from build123d import *

# Parameters (mm, degrees)
SCHIZZO1_W                     = 28
SCHIZZO1_H                     = 25
BASE_FLANGIA1_DEPTH            = 2
BORDO_FLANGIA1_STRIP_W         = 9.4732
BORDO_FLANGIA1_STRIP_H         = 2
BORDO_FLANGIA1_STRIP_CUT_DEPTH = 25
BORDO_FLANGIA1_DEPTH           = 25
SCHIZZO3_R                     = 4
SCHIZZO3_R_2                   = 1.5
TAGLIO_ESTRUSIONE1_DEPTH       = 40.714606885
SCHIZZO4_R                     = 1.5
SCHIZZO4_R_2                   = 4
TAGLIO_ESTRUSIONE2_DEPTH       = 47.917480751


# Sheet-metal steps are written as plain solids
with BuildPart() as part:
    # Schizzo1 → Base-Flangia1 (new body)
    with BuildSketch(Plane(origin=(0, 0, 0), x_dir=(1, 0, 0), z_dir=(0, 1, 0))):
        Rectangle(SCHIZZO1_W, SCHIZZO1_H)
    extrude(amount=BASE_FLANGIA1_DEPTH)

    # Bordo-Flangia1 strip (across the edge) → Bordo-Flangia1 strip cut (cut)
    with BuildSketch(Plane(origin=(-14, 2, -12.5), x_dir=(1, 0, 0), z_dir=(0, 0, 1))):
        with Locations((-2, -1)):
            Rectangle(BORDO_FLANGIA1_STRIP_W, BORDO_FLANGIA1_STRIP_H)
    extrude(amount=BORDO_FLANGIA1_STRIP_CUT_DEPTH, mode=Mode.SUBTRACT)

    # Bordo-Flangia1 section (across the edge) → Bordo-Flangia1 (add)
    with BuildSketch(Plane(origin=(-14, 2, -12.5), x_dir=(1, 0, 0), z_dir=(0, 0, 1))):
        with BuildLine():
            Line((0, 0.7366), (0, 35))
            Line((0, 35), (2, 35))
            Line((2, 35), (2, 0.7366))
            ThreePointArc((2, 0.7366), (2.215745145, 0.215745145), (2.7366, 0))
            Line((2.7366, 0), (2.7366, -2))
            ThreePointArc((2.7366, -2), (0.801531583, -1.198468417), (0, 0.7366))
        make_face()
    extrude(amount=BORDO_FLANGIA1_DEPTH)

    # Schizzo3 → Taglio-Estrusione1 (cut, through all)
    with BuildSketch(Plane(origin=(0, 2, 0), x_dir=(1, 0, 0), z_dir=(0, 1, 0))):
        with Locations(Location((1.5, 0, 0), (0, 0, 270))):
            Circle(SCHIZZO3_R)
        with Locations(Location((1.5, 7, 0), (0, 0, 270))):
            Circle(SCHIZZO3_R_2)
        with Locations(Location((-5.5, 0, 0), (0, 0, 270))):
            Circle(SCHIZZO3_R_2)
        with Locations(Location((1.5, -7, 0), (0, 0, 270))):
            Circle(SCHIZZO3_R_2)
        with Locations(Location((8.5, 0, 0), (0, 0, 270))):
            Circle(SCHIZZO3_R_2)
        with BuildLine():
            ThreePointArc((1.5, 12.5), (10.338834766, 8.838834764), (14, -3e-09))
            Line((14, -3e-09), (14, 12.5))
            Line((14, 12.5), (1.5, 12.5))
        make_face()
        with BuildLine():
            ThreePointArc((14, -3e-09), (10.338834764, -8.838834766), (1.5, -12.5))
            Line((1.5, -12.5), (14, -12.5))
            Line((14, -12.5), (14, -3e-09))
        make_face()
    extrude(amount=-TAGLIO_ESTRUSIONE1_DEPTH, mode=Mode.SUBTRACT)

    # Schizzo4 → Taglio-Estrusione2 (cut, through all)
    with BuildSketch(Plane(origin=(-12, 0, 0), x_dir=(0, 0, -1), z_dir=(1, 0, 0))):
        with BuildLine():
            Line((12.5, 24.5), (12.5, 37))
            Line((12.5, 37), (3.9e-08, 37))
            ThreePointArc((3.9e-08, 37), (8.838834779, 33.338834751), (12.5, 24.5))
        make_face()
        with BuildLine():
            ThreePointArc((-12.5, 24.5), (-8.838834751, 33.338834779), (3.9e-08, 37))
            Line((3.9e-08, 37), (-12.5, 37))
            Line((-12.5, 37), (-12.5, 24.5))
        make_face()
        with Locations(Location((0, 31.5, 0), (0, 0, 90))):
            Circle(SCHIZZO4_R)
        with Locations(Location((0, 24.5, 0), (0, 0, 90))):
            Circle(SCHIZZO4_R_2)
        with Locations(Location((7, 24.5, 0), (0, 0, 90))):
            Circle(SCHIZZO4_R)
        with Locations(Location((0, 17.5, 0), (0, 0, 90))):
            Circle(SCHIZZO4_R)
        with Locations(Location((-7, 24.5, 0), (0, 0, 90))):
            Circle(SCHIZZO4_R)
    extrude(amount=-TAGLIO_ESTRUSIONE2_DEPTH, mode=Mode.SUBTRACT)


solid = part.part
Can you work these out from the model? Positions are in its coordinate system, mm. A direction names the side the tool comes from. Give positions to 0.01 mm unless a question says otherwise; leave off trailing zeros. Loops run counter-clockwise (first coordinate to the right, second up) from the corner with the lowest first, then second, coordinate; pieces in that order, holes last. Notation, with made-up numbers: M 42,26.5 L 67,26.5 A11 ccw 67,32.5 Z; hole C 17,-6 d8. An arc over 180 degrees is marked long. One line per item, written item: value. Start each with the question number.
1) If we section it at A-A, the plane x = -5.5: Write out the boundary of the cut face in (y, z), and give its area (3 significant figures).
2) If we section it at B-B, the plane y = 17.5: Write out the boundary of the cut face in (x, z), and give its area (3 significant figures).
3) Thinking about a two-plate mould opening in Y: for faces 3 (the face through (-2, 0, -3)), 4 (the face through (1.57, 1.01, 5.5)), 5 (the face through (-13, 16, 0)), which applies, +Y half, -Y half, draft (parallel to the pull), parting line (faces both ways), or undercut?
4) On a 3-axis mill with a long thin cutter (end or side, diameter ignored), from which of +Z, -Z, +X, -X, +Y, -Y can I reach the whole of each face in a straight line? I mean faces 1 (the face through (-5.05, 1.01, 1.43)), 2 (the face through (-12, 20, 0)). Say none if no direction works.
5) If we section it at C-C, the plane z = 0.75: Give the number of separate pieces and of enclosed holes in the cut face, and give its area (3 significant figures).
6) If I drill on line 1 (Z direction, x = -13.4, y = 24.5); line 2 (Y direction, x = -0.75, z = 10.75); line 3 (X direction, y = 9, z = -0.5), over which ranges is the centre line in solid material (lowest first)? Write a range as [from, to].
7) I'm going to push flat-ended pins straight in: pin 1 (4 mm diameter, centred on x = 1.5, z = -7, fed in from -Y); pin 2 (12.5 mm diameter, centred on y = 28, z = -3, fed in from +X); pin 3 (6 mm diameter, centred on x = -1.5, z = -1.5, fed in from +Y). Where does each tip first touch, or does it pass through?
8) If we section it at D-D, the plane x = 0.75: Write out the boundary of the cut face in (y, z).
Completed:
1. outline: M 0,-12.5 L 2,-12.5 L 2,-1.5 L 0,-1.5 Z; M 0,1.5 L 2,1.5 L 2,12.5 L 0,12.5 Z
1. area: 44.0 mm^2
2. outline: M -14,-12.5 L -12,-12.5 L -12,-1.5 L -14,-1.5 Z; M -14,1.5 L -12,1.5 L -12,12.5 L -14,12.5 Z
2. area: 44.0 mm^2
3. face 3: -Y half
3. face 4: draft
3. face 5: undercut
4. face 1: +Y, -Y
4. face 2: +Z, -Z, +X, +Y
5. separate pieces: 7
5. enclosed holes: 0
5. area: 72.2 mm^2
6. line 1: z = [-12.5, -8.5], [-5.5, -4], [4, 5.5], [8.5, 12.5]
6. line 2: y = [0, 2]
6. line 3: x = [-14, -12]
7. pin 1: stops at y = 0
7. pin 2: stops at x = -12
7. pin 3: stops at y = 2
8. outline: M 0,-12.5 L 2,-12.5 L 2,-8.3 L 0,-8.3 Z; M 0,-5.7 L 2,-5.7 L 2,-3.93 L 0,-3.93 Z; M 0,3.93 L 2,3.93 L 2,5.7 L 0,5.7 Z; M 0,8.3 L 2,8.3 L 2,12.5 L 0,12.5 Z
